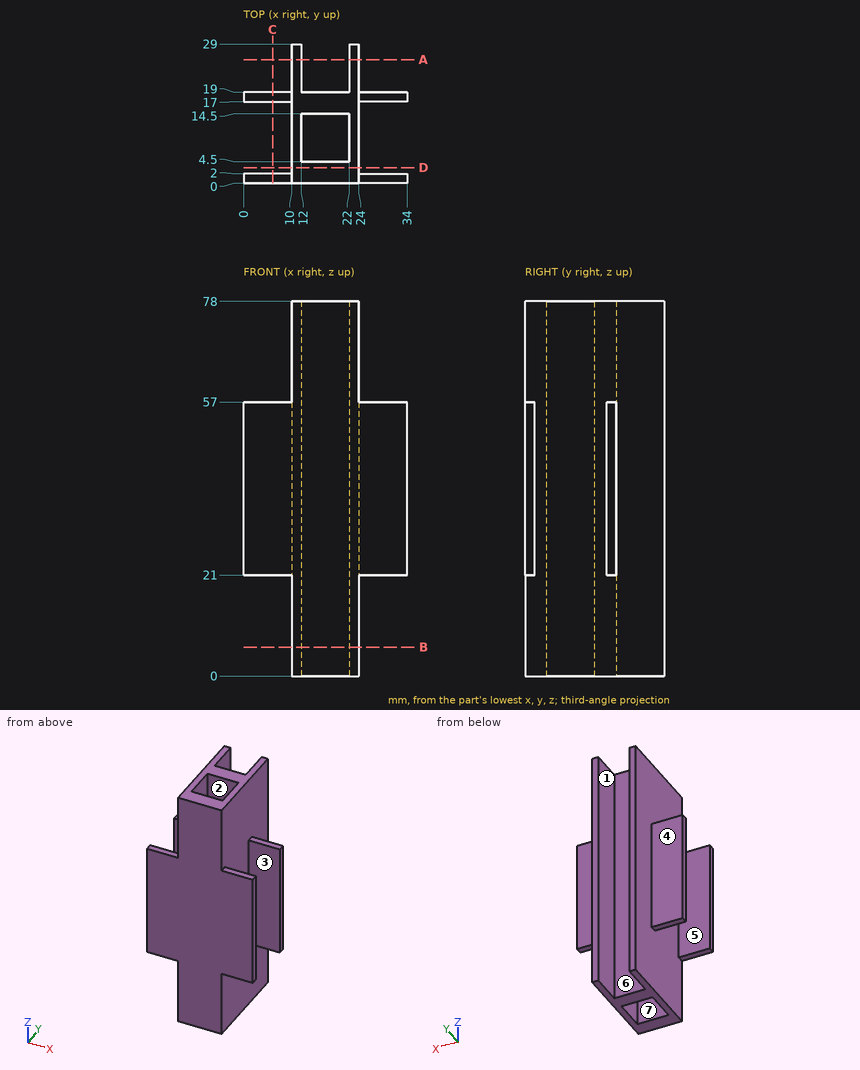
Design review of the part shown in the three views and the two pictorial views. Dimensions are in mm from the part's minimum x, y and z. A direction names the side the tool comes from. Give positions to 0.01 mm unless a question says otherwise; leave off trailing zeros. Order: outer loops, then holes, each group sorted by start corner. A loop starts at its lowest first (then second) coordinate and runs counter-clockwise, first axis right, second up. Notation, with made-up numbers: (87.25, 30.5) -> (92.25, 30.5) arc R25 ccw to (92.25, 69.5) -> close; hole circle Ø7 at (47, 31). An arc over 180 degrees is marked (long way). Write each question's results on one line, items separated by ' | '. Start each with the question number.
Q1. Mouldability with a two-part tool opening along Y and no side actions: class the marked faces 1, 2, 3 and 4 as +Y half, -Y half, draft (parallel to the pull), parting line (faces both ways), or undercut.
Q2. Add section C-C on x = 6. Give the boundary of the cut face in (y, z), and give its area (3 significant figures).
Q3. Add section D-D on y = 3.25. Give the boundary of the cut face in (x, z).
Q4. Machinability: for the marked faces 5, 6 and 7, which of the approach directions +Z, -Z, +X, -X, +Y, -Y give a long, thin tool a straight path to every point of the face, cutting with its end or side? Answer none if there is none.
Q5. Wall thickness on L1, parallel to Y at x = 1.5, z = 25.5; L2, parallel to X at y = 20.25, z = 36; L3, parallel to Y at x = 13, z = 5: over which ranges is each line inside the solid? List them lowest first. Write a range as from..to.
Q6. For pin 1 (5 mm diameter, centred on y = 6.5, z = 15, fed in from -X); pin 2 (5 mm diameter, centred on y = 9.5, z = 40.5, fed in from +X); pin 3 (3 mm diameter, centred on x = 29.5, z = 30.5, fed in from +Y), all flat-tipped, find the tip position at first contact; note any pin that passes through.
Q7. Add section A-A on y = 25.75. Give the boundary of the cut face in (x, z).
Q8. Add section B-B on z = 6. Give the boundary of the cut face in (x, y).
Found:
1) face 1: draft | face 2: undercut | face 3: undercut | face 4: +Y half
2) outline: (0, 21) -> (2, 21) -> (2, 57) -> (0, 57) -> close; (17, 21) -> (19, 21) -> (19, 57) -> (17, 57) -> close | area: 144 mm2
3) outline: (10, 0) -> (24, 0) -> (24, 78) -> (10, 78) -> close
4) face 5: +Z, -Z, -X | face 6: +Z, -Z, +Y | face 7: +Z, -Z
5) L1: y = 0..2, 17..19 | L2: x = 10..12, 22..24 | L3: y = 0..4.5, 14.5..19
6) pin 1: stops at x = 10 | pin 2: stops at x = 24 | pin 3: stops at y = 19
7) outline: (10, 0) -> (12, 0) -> (12, 78) -> (10, 78) -> close; (22, 0) -> (24, 0) -> (24, 78) -> (22, 78) -> close
8) outline: (10, 0) -> (24, 0) -> (24, 29) -> (22, 29) -> (22, 19) -> (12, 19) -> (12, 29) -> (10, 29) -> close; hole (12, 4.5) -> (22, 4.5) -> (22, 14.5) -> (12, 14.5) -> close
